Study the drawing (mm; zero at the part's minimum x, y, z) and answer. A direction names the side the tool comes from. Coordinates: 2 decimals unless noted, no trailing zeros. Write each loop counter-clockwise with the first axis right and the second up, starting at its lowest first coordinate (ties: lowest second). Pieces come first, ordered by that corner, then holes. Notation, with made-up numbers: (-27, 30) -> (1, 30) arc R15 cw to (1, 36) -> close; hole circle Ø11 at (5, -18.5). An arc over 180 degrees is marked (long way). Write item = value, one per line. Start each with the question number.
1) A tool of negligible diameter and unlimited length cuts with its end or side. For the marked faces 5, 6, 7 and 8, from which of +Z, -Z, +X, -X, +Y, -Y can it reach the whole face along a straight path? Write none if from no direction.
2) Find the intervals of material crossed by line 1 along X through (y, z) = (53, 19) (1 decimal); line 2 along Z through (x, y) = (7, 86) (1 decimal); line 3 along Y through (x, z) = (100.5, 28) (1 decimal), in increasing order. Write a range as from..to.
3) Section A-A (z = 43) is taken. Determine the outline of the cut face in (x, y) (1 decimal), plus the area to 3 significant figures.
4) Section B-B (z = 68) is taken. Determine the outline of the cut face in (x, y) (1 decimal).
5) Section D-D (y = 70.5) is taken. Count the separate pieces of the cut face and the enclosed holes in it, plus the area to 3 significant figures.
6) Section C-C (x = 102.5) is taken. Determine the outline of the cut face in (y, z) (1 decimal).
7) Flat-ended cylindrical pins translate along their axes: pin 1 Ø15.5 at (x, y) = (67.87, 67.87) entering from -Z; pin 2 Ø6 at (x, z) = (97, 30.5) entering from +Y; pin 3 Ø10.5 at (y, z) = (75.5, 62.5) entering from -X; pin 4 Ø1.5 at (x, y) = (118.5, 46.5) entering from +Z (1 decimal). Find the tip coordinate at first contact, or state that the pin passes through.
8) For a pull along Z with two mould halves and no side action, classify the marked faces 1, 2, 3 and 4 as released by +Z, released by -Z, zero draft, split by the parting line, or undercut.
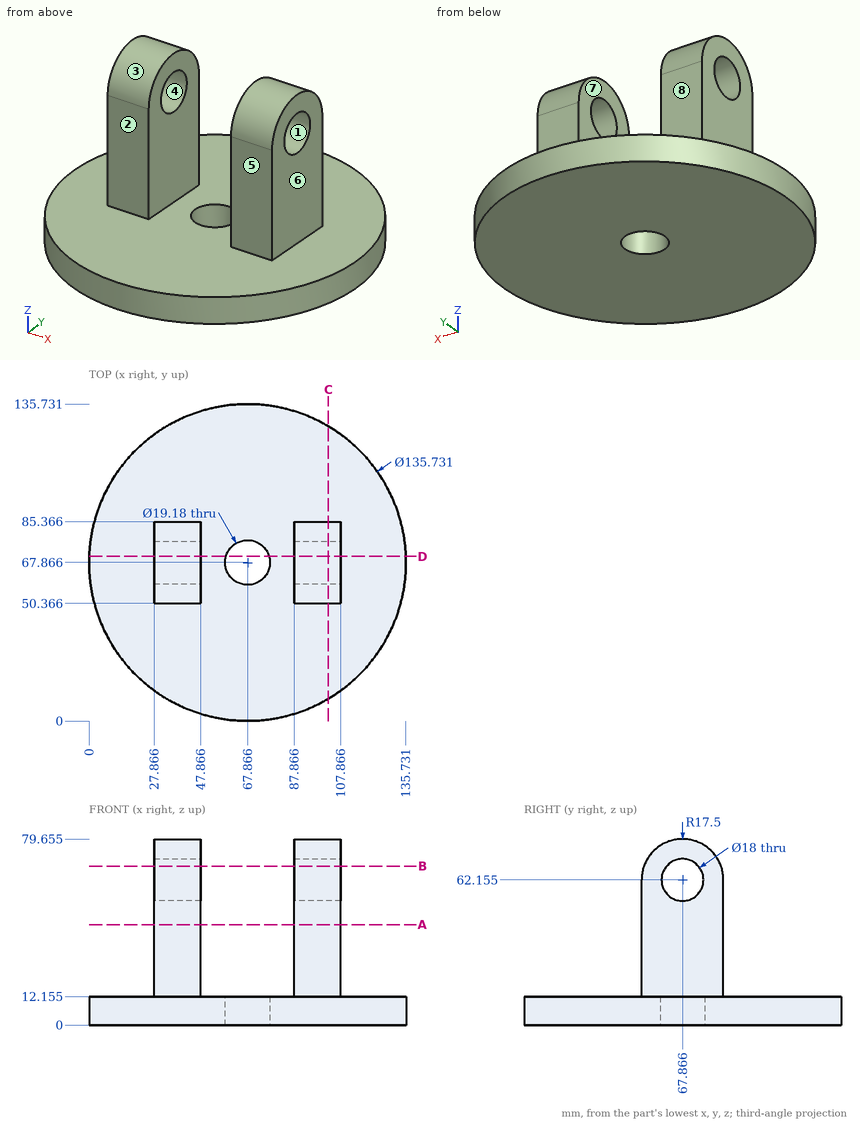
Answer key:
q1.face_5 = +Z, +X, -X, -Y
q1.face_6 = +Z, +X, +Y, -Y
q1.face_7 = +Z, +Y, -Y
q1.face_8 = +Z, +X, -X, +Y
q2.line_1 = 27.9..47.9, 87.9..107.9
q2.line_2 = 0..12.2
q2.line_3 = 50.4..85.4
q3.outline = (27.9, 50.4) -> (47.9, 50.4) -> (47.9, 85.4) -> (27.9, 85.4) -> close; (87.9, 50.4) -> (107.9, 50.4) -> (107.9, 85.4) -> (87.9, 85.4) -> close
q3.area = 1,400 mm^2
q4.outline = (27.9, 51.4) -> (47.9, 51.4) -> (47.9, 61) -> (27.9, 61) -> close; (27.9, 74.7) -> (47.9, 74.7) -> (47.9, 84.4) -> (27.9, 84.4) -> close; (87.9, 51.4) -> (107.9, 51.4) -> (107.9, 61) -> (87.9, 61) -> close; (87.9, 74.7) -> (107.9, 74.7) -> (107.9, 84.4) -> (87.9, 84.4) -> close
q5.separate_pieces = 4
q5.enclosed_holes = 0
q5.area = 3,430 mm^2
q6.outline = (9.5, 0) -> (126.2, 0) -> (126.2, 12.2) -> (85.4, 12.2) -> (85.4, 62.2) arc R17.5 ccw to (50.4, 62.2) -> (50.4, 12.2) -> (9.5, 12.2) -> close; hole circle Ø18 at (67.9, 62.2)
q7.pin_1 = through
q7.pin_2 = 85.37
q7.pin_3 = 27.87
q7.pin_4 = 12.2
q8.face_1 = undercut
q8.face_2 = zero draft
q8.face_3 = released by +Z
q8.face_4 = undercut
